Geometry: see drawing. Coordinates: mm, zero at the bounding-box minimum. A direction names the side the tool comes from. Give positions to 0.01 mm unless a question says otherwise; leave off trailing zeros. Loops run counter-clockwise (first coordinate to the right, second up) from the corner with the lowest first, then second, coordinate; pieces in that order, holes last. Notation, with made-up numbers: M 49,47 L 70,47 A25 ccw 70,78 Z; hole C -24,50.5 d3. An arc over 180 degrees is marked long. Put each result on its own line as item: value.
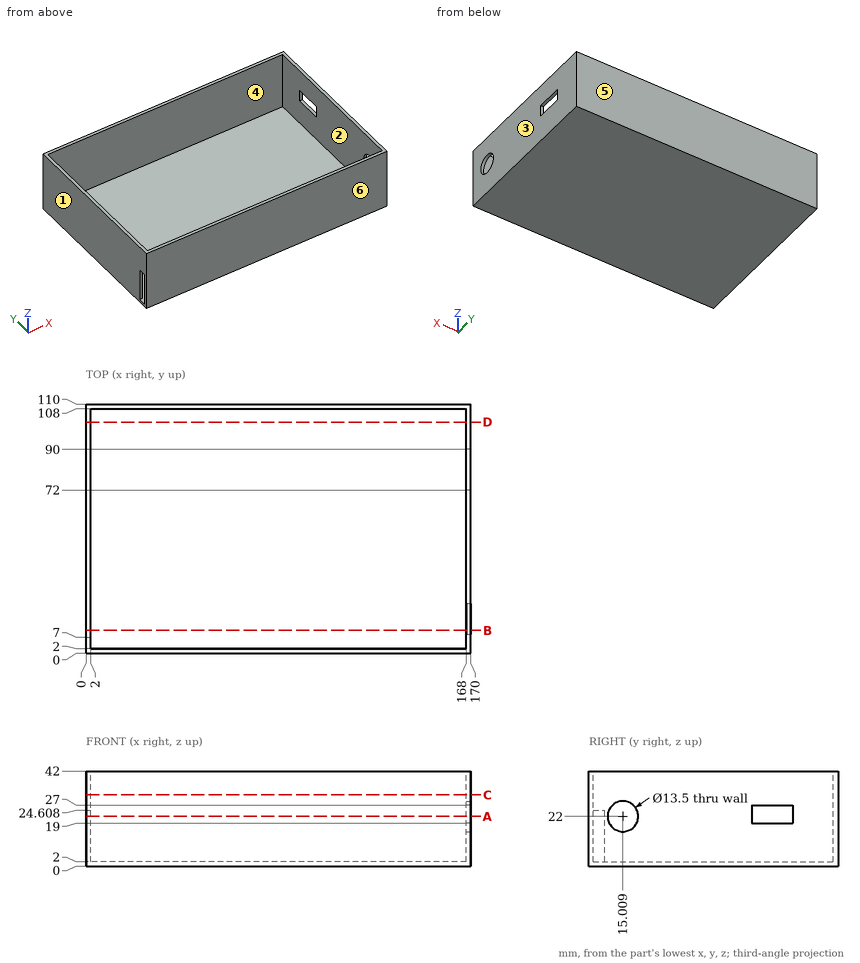
Item 1: Mould query, pull axis Y, two halves, no side actions, for the marked faces 3, 4, 5 and 6. Classes: pulls with the +Y half, pulls with the -Y half, needs draft (parallel to the pull), parting line crosses it, or undercut.
Output values:
face 3: needs draft
face 4: undercut
face 5: pulls with the +Y half
face 6: pulls with the -Y half
Item 2: Set-up query: the marked faces 1 and 2. Return all of +Z, -Z, +X, -X, +Y, -Y with unobstructed straight access to the full face (end or side cutting, diameter ignored); none if empty.
Output values:
face 1: +Z, -Z, -X, +Y, -Y
face 2: +Z
Item 3: Section A-A on z = 22. Output: boundary loops of the cut face in (x, y).
Output values:
outline: M 0,0 L 170,0 L 170,8.26 L 168,8.26 L 168,2 L 0,2 Z; M 0,7 L 2,7 L 2,108 L 168,108 L 168,90 L 170,90 L 170,110 L 0,110 Z; M 168,21.76 L 170,21.76 L 170,72 L 168,72 Z
Item 4: Section D-D on y = 102. Output: boundary loops of the cut face in (x, z).
Output values:
outline: M 0,0 L 170,0 L 170,42 L 168,42 L 168,2 L 2,2 L 2,42 L 0,42 Z
Item 5: Pin query (flat end, axial travel): pin 1 Ø10 at (x, y) = (87, 69.5) entering from +Z. Return the tip coordinate at first contact, or that it passes through.
Output values:
pin 1: z = 2
Item 6: Section B-B on y = 10. Output: boundary loops of the cut face in (x, z) (1 decimal), then the cut area to 3 significant figures.
Output values:
outline: M 0,0 L 170,0 L 170,17.5 L 168,17.5 L 168,2 L 2,2 L 2,42 L 0,42 Z; M 168,26.5 L 170,26.5 L 170,42 L 168,42 Z
area: 482 mm²
Item 7: Line query: probe 1 along X at (y, z) = (49, 18); probe 2 along Y at (x, z) = (45.5, 6); probe 3 along Z at (x, y) = (75, 24.5). Output: solid intervals per line, ascending. Write a range as [from, to].
Output values:
probe 1: [0, 2], [168, 170]
probe 2: [0, 2], [108, 110]
probe 3: [0, 2]
Item 8: Section C-C on z = 31.5. Output: boundary loops of the cut face in (x, y), then the cut area to 3 significant figures.
Output values:
outline: M 0,0 L 170,0 L 170,110 L 0,110 Z; hole M 2,2 L 168,2 L 168,108 L 2,108 Z
area: 1,100 mm²
